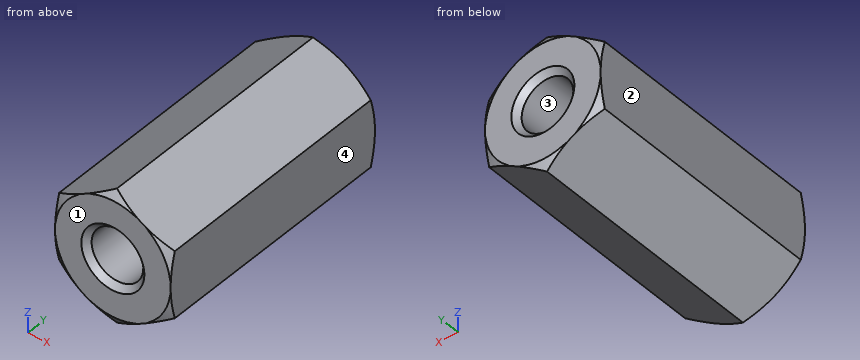
Autodesk Inventor part; units mm, degrees
ref_plane "YZ Plane" through (0, 0, 0) normal (1, 0, 0) x (0, 1, 0)
ref_plane "XZ Plane" through (0, 0, 0) normal (0, 1, 0) x (-1, 0, 0)
ref_plane "XY Plane" through (0, 0, 0) normal (0, 0, 1) x (1, 0, 0)
sketch "スケッチ1" plane through (0, 0, 0) normal (1, 0, 0) x (0, 1, 0)
  line L0 (-6, 0) -> (6, 0)
  line L1 (0, 0) -> (0, 3.1754) construction
  line L2 (-5.7544, 3.1754) -> (-6, 2.75)
  line L3 (-6, 2.75) -> (-6, 0)
  line L4 (-5.7544, 3.1754) -> (5.7544, 3.1754)
  line L5 (5.7544, 3.1754) -> (6, 2.75)
  line L6 (6, 2.75) -> (6, 0)
  dimension "d1" = 2.75
  dimension "d2" = 3.1754
  dimension "d3" = 30
  dimension "d4" = 12
revolve "回転1" add sketch "スケッチ1" angle 360 about axis through (0, -6, 0) along (0, 1, 0)
sketch "スケッチ2" plane through (0, 6, 0) normal (0, 1, 0) x (1, 0, 0)
  circle A0 centre (0, 0) radius 3.1754
  line L0 (0, -3.1754) -> (-2.75, -1.5877)
  line L1 (-2.75, -1.5877) -> (-2.75, 1.5877)
  line L2 (-2.75, 1.5877) -> (0, 3.1754)
  line L3 (0, 3.1754) -> (2.75, 1.5877)
  line L4 (2.75, 1.5877) -> (2.75, -1.5877)
  line L5 (2.75, -1.5877) -> (0, -3.1754)
  point P0 (0, 0)
  point P1 (0, 0)
  point P2 (2.75, -1.5877)
  point P3 (2.75, -1.5877)
  point P4 (2.75, 1.5877)
  point P5 (2.75, 1.5877)
  point P6 (0, 3.1754)
  point P7 (0, 3.1754)
  point P8 (-2.75, 1.5877)
  point P9 (-2.75, 1.5877)
  point P10 (-2.75, -1.5877)
  point P11 (-2.75, -1.5877)
extrude "押し出し1" cut sketch "スケッチ2" against normal through all contours A0 L4 | L3 A0 | A0 L5 | L2 A0 | A0 L0 | L1 A0
hole "穴1" at (0, 6, 0) direction (0, -1, 0) diameter 2.459 end through all countersink diameter 3 countersink angle 90
mirror "ミラー1" about plane through (0, 0, 0) normal (0, 1, 0) of "穴1"
equation "\"d2\" = 1.1547 * d1"
properties part number "ASL-312BE" material "アルミニウム 2014-T4"
Can you work these out from the model? Positions are in its coordinate system, mm. Face numbers are marked on the shaded views. Give positions to 0.01 mm unless a question says otherwise; leave off trailing zeros. Loops run counter-clockwise (first coordinate to the right, second up) from the corner with the lowest first, then second, coordinate; pieces in that order, holes last. Notation, with made-up numbers: M 77,70 L 119,70 A19 ccw 119,100 Z; hole C -22,25.25 d7. An arc over 180 degrees is marked long. One line per question, with ' | ' between items. Start each with the question number.
Q1. For pin 1 Ø1 at (y, z) = (-1.5, -2.5) entering from -X, with a flat end and sliding along its axis, tell me the tip position at first contact or that it passes through.
Q2. If we mould it in two halves opening along X, with no side actions, what happens to the marked faces 1, 2, 3 and 4? For each: +X half, -X half, draft (parallel to the pull), parting line (faces both ways), or undercut.
Q3. If I drill on line 1 (X direction, y = -2.25, z = 0); line 2 (Z direction, x = -0.95, y = 1); line 3 (Y direction, x = -0.1, z = 2.75), over which ranges is the centre line in solid material (lowest first)? Write a range as from..to.
Q4. If we section it at A-A (y = -0.5): Please give me the cut outline in (x, z).
Computed:
1) pin 1: stops at x = -2.04
2) face 1: draft | face 2: -X half | face 3: undercut | face 4: +X half
3) line 1: x = -2.75..-1.23, 1.23..2.75 | line 2: z = -2.63..-0.78, 0.78..2.63 | line 3: y = -6..6
4) outline: M -2.75,-1.59 L 0,-3.18 L 2.75,-1.59 L 2.75,1.59 L 0,3.18 L -2.75,1.59 Z; hole C 0,0 d2.46
